Answer from the drawing. Dimensions are ordinates in mm from the lowest x, y and z of the part. A direction names the side the tool comes from. Give positions to 0.01 mm unless a question says otherwise; leave off trailing zeros. Loops run counter-clockwise (first coordinate to the right, second up) from the corner with the lowest first, then second, coordinate; pieces in that order, holes last. Notation, with made-up numbers: (-11.5, 60) - (0.5, 60) arc R15 ccw to (0.5, 76) - close; hole circle Ø9 at (73, -31). An arc over 180 degrees is marked (long way). Write each question's results on one line, items separated by ' | '. Start each with the question number.
Q1. The part is cut by section C-C, the plane y = 30. State how many separate pieces and enclosed holes the cut face has, plus the area to 3 significant figures.
Q2. The part is cut by section B-B, the plane x = 12. Write down the section's boundary in (y, z), plus the area to 3 significant figures.
Q3. The part is cut by section D-D, the plane x = 95. Write down the section's boundary in (y, z).
Q4. For the marked faces 4, 5 and 6, determine the directions among +Z, -Z, +X, -X, +Y, -Y from which every point of the face is accessible in a straight line to the end or side of a thin tool.
Q5. Determine the mould class of the marked faces 1, 2 and 3 for opening direction X: +X half, -X half, draft (parallel to the pull), parting line (faces both ways), or undercut.
Q6. The part is cut by section A-A, the plane z = 44. Write down the section's boundary in (x, y).
Q7. Find the intervals of material crossed by line 1 (Z direction, x = 151.65, y = 30); line 2 (X direction, y = 32, z = 88.5); line 3 (Z direction, x = 46, y = 15) (1 decimal), in increasing order. Write a range as from..to.
Q8. Given pin 1 (19 mm diameter, centred on x = 179.58, y = 48, fed in from -Z); pin 2 (9 mm diameter, centred on y = 12.36, z = 36.43, fed in from -X); pin 3 (5 mm diameter, centred on y = 48, z = 114, fed in from +X), each flat-ended and moving along its own axis, determine where each tip first touches the part or whether it passes through.
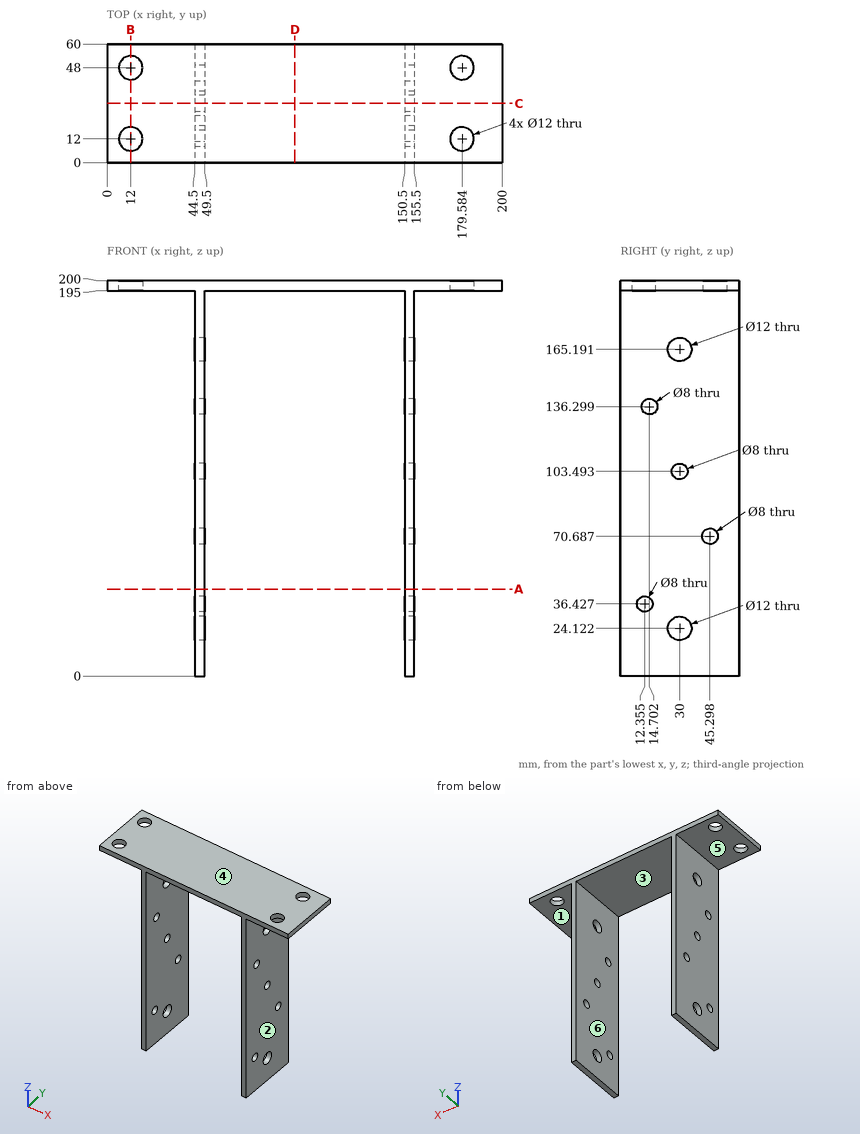
Check sheet entries:
1) separate pieces: 7 | enclosed holes: 0 | area: 2,630 mm^2
2) outline: (0, 195) - (6, 195) - (6, 200) - (0, 200) - close; (18, 195) - (42, 195) - (42, 200) - (18, 200) - close; (54, 195) - (60, 195) - (60, 200) - (54, 200) - close | area: 180 mm^2
3) outline: (0, 195) - (60, 195) - (60, 200) - (0, 200) - close
4) face 4: +Z, +X, -X, +Y, -Y | face 5: -Z, -X, +Y, -Y | face 6: -Z, +Y, -Y
5) face 1: draft | face 2: +X half | face 3: undercut
6) outline: (44.5, 0) - (49.5, 0) - (49.5, 60) - (44.5, 60) - close; (150.5, 0) - (155.5, 0) - (155.5, 60) - (150.5, 60) - close
7) line 1: z = 0..18.12, 30.12..99.49, 107.49..159.19, 171.19..200 | line 2: x = 44.5..49.5, 150.5..155.5 | line 3: z = 0..33.4, 39.4..132.3, 140.3..200
8) pin 1: stops at z = 195 | pin 2: stops at x = 44.5 | pin 3: stops at x = 155.5
